Autodesk Inventor part; units mm, degrees
ref_plane "YZ Plane" through (0, 0, 0) normal (1, 0, 0) x (0, 1, 0)
ref_plane "XZ Plane" through (0, 0, 0) normal (0, 1, 0) x (-1, 0, 0)
ref_plane "XY Plane" through (0, 0, 0) normal (0, 0, 1) x (1, 0, 0)
sketch "Sketch1" plane through (0, 0, 0) normal (0, 0, 1) x (1, 0, 0)
  line L0 (12.1296, 191.2771) -> (12.1296, 1.2771)
  line L1 (12.1296, 1.2771) -> (32.1296, 1.2771)
  line L2 (12.1296, 191.2771) -> (32.1296, 189.5273)
  line L3 (12.1296, 191.2771) -> (39.6219, 191.2771) construction
  line L4 (32.1296, 1.2771) -> (32.1296, 189.5273)
  point P0 (0, 0)
  dimension "d0" = 190
  dimension "d1" = 20
  dimension "d2" = 5
extrude "Extrusion1" add sketch "Sketch1" along normal mid plane 10
sketch "Sketch2" plane through (12.1296, 191.2771, 5) normal (0.0871557, 0.9961947, 0) x (0.9961947, -0.0871557, 0)
  circle A0 centre (9.4291, 5) radius 2.5
  point P0 (4.5875, 5)
  dimension "d7" = 5
extrude "Extrusion2" add sketch "Sketch2" along normal blind 2
properties part number "stand2"
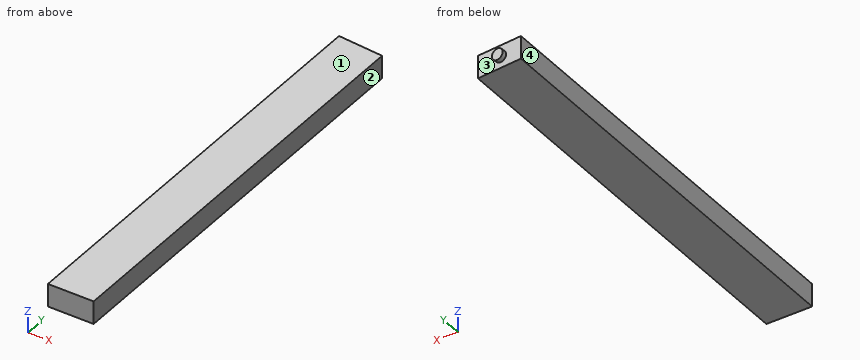
Source: CAD feature listing. Evaluate the final solid. Frame: model axes, mm. Face numbers are marked on the shaded views. Give positions to 0.01 mm unless a question says otherwise; leave off trailing zeros. Loops run counter-clockwise (first coordinate to the right, second up) from the corner with the lowest first, then second, coordinate; pieces in that order, holes last. Notation, with made-up numbers: (-5.5, 87) - (37.5, 87) arc R34 ccw to (37.5, 123) - close; hole circle Ø1 at (88.5, 82.5). An arc over 180 degrees is marked (long way). Use CSV: the item, a comma, the result in double quotes. Start each with the question number.
1. Ray query, L1, parallel to Y at x = 25, z = -3.5; L2, parallel to Y at x = 20, z = 4. Return the intervals inside material, ascending.
2. Draft query along X for the marked faces 1, 2, 3 and 4. Return one class per face: +X half, -X half, draft (parallel to the pull), parting line (faces both ways), or undercut.
3. Section A-A (x = 30). Output: boundary loops of the cut face in (y, z).
Response:
1,L1,"1.28 to 190.15"
1,L2,"1.28 to 190.59"
2,face 1,"draft"
2,face 2,"+X half"
2,face 3,"undercut"
2,face 4,"-X half"
3,outline,"(1.28, -5) - (189.71, -5) - (189.71, 5) - (1.28, 5) - close"
